Check sheet for the modelled part. Datum: model origin and axes. Units: mm. Face numbers are marked on the shaded views. A direction names the side the tool comes from. Give positions to 0.01 mm unless a question says otherwise; leave off trailing zeros. Order: outer loops, then holes, each group sorted by start corner. A loop starts at its lowest first (then second) coordinate and runs counter-clockwise, first axis right, second up. Notation, with made-up numbers: (68, -37.75) -> (97, -37.75) arc R17 ccw to (97, -24.75) -> close; hole circle Ø3 at (1.25, 30.5). An arc over 180 degrees is marked (long way). One line per question, with ' | ' between items.
Autodesk Inventor part; units mm, degrees
ref_plane "YZ Plane" through (0, 0, 0) normal (1, 0, 0) x (0, 1, 0)
ref_plane "XZ Plane" through (0, 0, 0) normal (0, 1, 0) x (-1, 0, 0)
ref_plane "XY Plane" through (0, 0, 0) normal (0, 0, 1) x (1, 0, 0)
sketch "Sketch1" plane through (0, 0, 0) normal (0, 0, 1) x (1, 0, 0)
  circle A0 centre (0, 0) radius 6.1
  line L0 (-12.5, -10) -> (12.5, -10)
  line L1 (12.5, -10) -> (12.5, 10)
  line L2 (12.5, 10) -> (-12.5, 10)
  line L3 (-12.5, 10) -> (-12.5, -10)
  line L4 (-12.5, -10) -> (12.5, 10) construction
  line L5 (12.5, -10) -> (-12.5, 10) construction
  dimension "d0" = 12.2
  dimension "d1" = 25
  dimension "d2" = 20
extrude "Extrusion1" add sketch "Sketch1" along normal blind 20
sketch "Sketch2" plane through (-12.5, 10, 0) normal (0, 1, 0) x (1, 0, 0)
  line L0 (0, 0) -> (0, -20) construction
  line L1 (25, -20) -> (0, -20) construction
  line L2 (0, 0) -> (25, -20) construction
  line L3 (0, -20) -> (25, 0) construction
  circle A0 centre (12.5, -10) radius 1
  point P0 (12.5, 0)
  dimension "d5" = 2
extrude "Extrusion2" cut sketch "Sketch2" against normal blind 100
sketch "Sketch3" plane through (-12.5, 10, 0) normal (0, 1, 0) x (1, 0, 0)
  circle A0 centre (12.5, -10) radius 1
  line L0 (25, 0) -> (0, 0)
  line L1 (0, 0) -> (0, -20)
  line L2 (25, -20) -> (0, -20)
  line L3 (25, 0) -> (25, -20)
  circle A1 centre (12.5, -10) radius 7.5
  point P0 (12.5, 0)
  dimension "d8" = 15
extrude "Extrusion3" add sketch "Sketch3" along normal blind 15 contours A1
sketch "Sketch4" plane through (-12.5, -10, 0) normal (0, -1, 0) x (1, 0, 0)
  line L0 (32.5, 25) -> (-7.5, 25)
  line L1 (-7.5, 25) -> (-7.5, -5)
  line L2 (-7.5, -5) -> (32.5, -5)
  line L3 (32.5, -5) -> (32.5, 25)
  circle A0 centre (12.5, 10) radius 1
  line L4 (32.5, 25) -> (-7.5, -5) construction
  line L5 (-7.5, 25) -> (32.5, -5) construction
  point P0 (12.5, 0)
  dimension "d11" = 30
  dimension "d12" = 40
extrude "Extrusion4" add sketch "Sketch4" along normal blind 3
properties part number "Arm_clip_template"
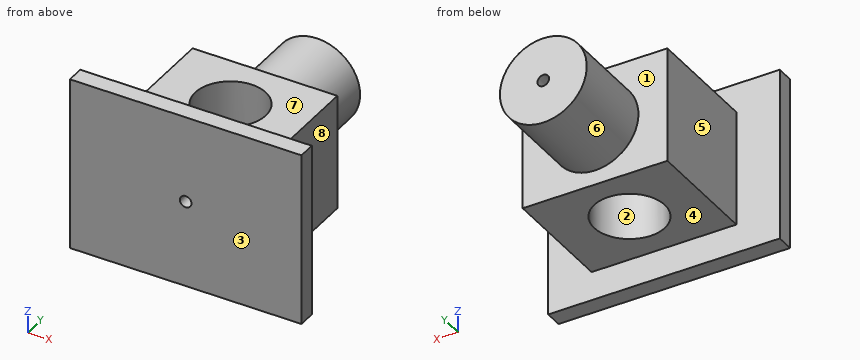
Q1. Section check A-A (z = 10). Enter the section's corners in (x, y).
Result sheet:
outline: (-20, -13) -> (-1, -13) -> (-1, -6.02) arc R6.1 cw to (-1, 6.02) -> (-1, 25) -> (-7.5, 25) -> (-7.5, 10) -> (-12.5, 10) -> (-12.5, -10) -> (-20, -10) -> close; (1, -13) -> (20, -13) -> (20, -10) -> (12.5, -10) -> (12.5, 10) -> (7.5, 10) -> (7.5, 25) -> (1, 25) -> (1, 6.02) arc R6.1 cw to (1, -6.02) -> close
Q2. Access from +Z, -Z, +X, -X, +Y, -Y to the whole of each face (thin tool, end or side, straight path). Record for the marked faces 4, 5, 6, 7 and 8.
Result sheet:
face 4: -Z, +X, -X, +Y | face 5: +Z, -Z, -X, +Y | face 6: +Y | face 7: +Z, +X, -X, +Y | face 8: +Z, -Z, +X, +Y
Q3. Section check C-C (y = 0). Enter the section's corners in (x, z), and give its area (3 significant figures).
Result sheet:
outline: (-12.5, 0) -> (-6.1, 0) -> (-6.1, 20) -> (-12.5, 20) -> close; (6.1, 0) -> (12.5, 0) -> (12.5, 20) -> (6.1, 20) -> close | area: 256 mm2
Q4. Depth check by flat-ended pin: pin 1 Ø12 at (x, y) = (2, -5.5) entering from +Z; pin 2 Ø2 at (y, z) = (-1.5, 1) entering from -X; pin 3 Ø5 at (x, y) = (-4.5, 17) entering from +Z; pin 4 Ø1 at (x, y) = (-10.5, 5) entering from +Z. Enter the tip coordinate at first touch or a pass-through.
Result sheet:
pin 1: stops at z = 25 | pin 2: stops at x = -12.5 | pin 3: stops at z = 17.23 | pin 4: stops at z = 20
Q5. Section check D-D (x = 5.5). Enter the section's corners in (y, z).
Result sheet:
outline: (-13, -5) -> (-10, -5) -> (-10, 0) -> (-2.64, 0) -> (-2.64, 20) -> (-10, 20) -> (-10, 25) -> (-13, 25) -> close; (2.64, 0) -> (10, 0) -> (10, 4.9) -> (25, 4.9) -> (25, 15.1) -> (10, 15.1) -> (10, 20) -> (2.64, 20) -> close
Q6. Mould release check, pull along Y, two halves, no side actions. Record for the marked faces 1, 2 and 3: pulls with the +Y half, pulls with the -Y half, needs draft (parallel to the pull), parting line crosses it, or undercut.
Result sheet:
face 1: pulls with the +Y half | face 2: undercut | face 3: pulls with the -Y half
Q7. Thickness scan on line 1 (Y direction, x = 0, z = 7); line 2 (Y direction, x = 1, z = 4); line 3 (Z direction, x = 0, y = -9). Record the ranges inside material, lowest first.
Result sheet:
line 1: y = -13 to -6.1, 6.1 to 25 | line 2: y = -13 to -6.02, 6.02 to 25 | line 3: z = 0 to 9, 11 to 20
Q8. Section check B-B (x = 0). Enter the section's corners in (y, z).
Result sheet:
outline: (-13, -5) -> (-10, -5) -> (-10, 0) -> (-6.1, 0) -> (-6.1, 9) -> (-13, 9) -> close; (-13, 11) -> (-6.1, 11) -> (-6.1, 20) -> (-10, 20) -> (-10, 25) -> (-13, 25) -> close; (6.1, 0) -> (10, 0) -> (10, 2.5) -> (25, 2.5) -> (25, 9) -> (6.1, 9) -> close; (6.1, 11) -> (25, 11) -> (25, 17.5) -> (10, 17.5) -> (10, 20) -> (6.1, 20) -> close
